```python
from build123d import *

# Parameters (mm, degrees)
SKETCH1_R                = 27.5
SKETCH1_R_2              = 2.5
BOSS_EXTRUDE1_DEPTH      = 10.5
SKETCH2_R                = 4
SKETCH2_R_2              = 2.5
BOSS_EXTRUDE2_DEPTH      = 11
SKETCH3_R                = 5
SKETCH3_R_2              = 4
BOSS_EXTRUDE3_DEPTH      = 1.5
BOSS_EXTRUDE4_DEPTH      = 11
FILLET2_R                = 0.5
FILLET5_R                = 1.5
CIRPATTERN1_COUNT        = 3
FILLET2_OF_CIRPATTERN1_R = 0.5
FILLET5_OF_CIRPATTERN1_R = 1.5
SKETCH5_R                = 1.5
CUT_EXTRUDE1_DEPTH       = 45.438159278
SKETCH6_R                = 2.75
CUT_EXTRUDE2_DEPTH       = 3
SKETCH7_R                = 4.25
CUT_EXTRUDE3_DEPTH       = 5
CIRPATTERN2_COUNT        = 3
CHAMFER1_SIZE            = 0.5
SKETCH9_R                = 8
CUT_EXTRUDE4_DEPTH       = 41.416580756
BOSS_EXTRUDE7_START      = -5.5
SKETCH10_R               = 8
SKETCH10_R_2             = 6.5
BOSS_EXTRUDE7_DEPTH      = 5.5
CHAMFER2_SIZE            = 0.5
BOSS_EXTRUDE8_START      = -1.5
SKETCH11_R               = 29
SKETCH11_R_2             = 27.5
BOSS_EXTRUDE8_DEPTH      = 1.5


with BuildPart() as part:
    # Sketch1 → Boss-Extrude1 (new body)
    with BuildSketch(Plane.XY):
        with Locations(Location((0, 0, 0), (0, 0, 180))):
            Circle(SKETCH1_R)
        with Locations(Location((0, 22.05, 0), (0, 0, 180))):
            Circle(SKETCH1_R_2, mode=Mode.SUBTRACT)
        with Locations(Location((19.095860153, -11.025, 0), (0, 0, 180))):
            Circle(SKETCH1_R_2, mode=Mode.SUBTRACT)
        with Locations(Location((-19.095860153, -11.025, 0), (0, 0, 180))):
            Circle(SKETCH1_R_2, mode=Mode.SUBTRACT)
    extrude(amount=BOSS_EXTRUDE1_DEPTH)

    # Sketch2 → Boss-Extrude2 (add)
    with BuildSketch(Plane.XY.offset(10.5)):
        with Locations((0, 22.05)):
            Circle(SKETCH2_R)
        with Locations(Location((0, 22.05, 0), (0, 0, 180))):
            Circle(SKETCH2_R_2, mode=Mode.SUBTRACT)
    boss_extrude2 = extrude(amount=BOSS_EXTRUDE2_DEPTH)

    # Sketch3 → Boss-Extrude3 (add)
    with BuildSketch(Plane.XY.offset(10.5)):
        with Locations((0, 22.05)):
            Circle(SKETCH3_R)
        with Locations((0, 22.05)):
            Circle(SKETCH3_R_2, mode=Mode.SUBTRACT)
    boss_extrude3 = extrude(amount=BOSS_EXTRUDE3_DEPTH)

    # Sketch4 → Boss-Extrude4 (add)
    with BuildSketch(Plane.XY.offset(10.5)):
        with BuildLine():
            ThreePointArc((-8.731428479, 7.173015873), (-14.812140242, 13.209015809), (-17.238712835, 21.426077098))
            ThreePointArc((-17.238712835, 21.426077098), (-23.815698604, 13.75), (-27.174883487, 4.216124695))
            ThreePointArc((-27.174883487, 4.216124695), (-18.845413371, 6.223181829), (-10.577728207, 3.975130938))
            ThreePointArc((-10.577728207, 3.975130938), (-9.786087063, 5.65), (-8.731428479, 7.173015873))
        make_face()
    boss_extrude4 = extrude(amount=BOSS_EXTRUDE4_DEPTH)

    # Fillet2
    fillet2_edges = [part.edges().sort_by_distance(p)[0] for p in [
        (-5, 22.05, 12),
    ]]
    fillet(fillet2_edges, radius=FILLET2_R)

    # Fillet5
    # the kernel refuses this fillet: 1.5 mm, written as the material it takes off along each edge
    with BuildSketch(Plane(origin=(-17.238712835, 21.426077098, 10.5), x_dir=(0.11627707658946446, -0.9932168149300573, 0), z_dir=(0, 0, 1))) as fillet5_piece_1:
        with BuildLine():
            CenterArc((2.88996817, -1.495158903), FILLET5_R, 94.604481761, 123.727317632)
            ThreePointArc((1.713319765, -2.425480639), (0.8238966, -1.235883765), (0, 0))
            ThreePointArc((0, 0), (1.384776415, -0.055672613), (2.769552829, 0))
        make_face()
    extrude(amount=18.423956554, mode=Mode.SUBTRACT)
    with BuildSketch(Plane(origin=(-27.174883487, 4.216124695, 10.5), x_dir=(0.9182895314900276, 0.39590950526076735, 0), z_dir=(0, 0, 1))) as fillet5_piece_2:
        with BuildLine():
            CenterArc((2.88996817, 1.495158903), FILLET5_R, 141.668200607, 123.727317632)
            ThreePointArc((1.713319765, 2.425480639), (0.8238966, 1.235883765), (0, 0))
            ThreePointArc((0, 0), (1.384776415, 0.055672613), (2.769552829, 0))
        make_face()
    extrude(amount=18.423956554, mode=Mode.SUBTRACT)
    with BuildSketch(Plane(origin=(-10.577728207, 3.975130938, 10.5), x_dir=(-0.8902885516550605, 0.4553968541743943, 0), z_dir=(0, 0, 1))) as fillet5_piece_3:
        with BuildLine():
            CenterArc((1.570607816, -1.498571769), FILLET5_R, 92.500493645, 86.512353367)
            ThreePointArc((0.070830441, -1.472729442), (0.059461178, -0.735208239), (0, 0))
            ThreePointArc((0, 0), (0.752582912, -0.016424661), (1.505165824, 0))
        make_face()
    extrude(amount=14.762914559, mode=Mode.SUBTRACT)
    with BuildSketch(Plane(origin=(-8.731428479, 7.173015873, 10.5), x_dir=(-0.5830170750372249, -0.8124599006812822, 0), z_dir=(0, 0, 1))) as fillet5_piece_4:
        with BuildLine():
            CenterArc((1.572292256, -1.496804369), FILLET5_R, 93.740653048, 86.512353367)
            ThreePointArc((0.07230688, -1.50342804), (0.052559138, -0.750924993), (0, 0))
            ThreePointArc((0, 0), (0.737215871, -0.024073752), (1.474431742, 0))
        make_face()
    extrude(amount=14.762914559, mode=Mode.SUBTRACT)

    # CirPattern1: Boss-Extrude2, Boss-Extrude3, Boss-Extrude4 ×3 about axis
    cirpattern1_axis = Axis((0, 0, 0), (0, 0, 1))
    add([boss_extrude2.rotate(cirpattern1_axis, i * 360 / CIRPATTERN1_COUNT) for i in range(1, CIRPATTERN1_COUNT)])
    add([boss_extrude3.rotate(cirpattern1_axis, i * 360 / CIRPATTERN1_COUNT) for i in range(1, CIRPATTERN1_COUNT)])
    add([boss_extrude4.rotate(cirpattern1_axis, i * 360 / CIRPATTERN1_COUNT) for i in range(1, CIRPATTERN1_COUNT)])

    # Fillet2 of CirPattern1
    fillet2_of_cirpattern1_edges = [part.edges().sort_by_distance(p)[0] for p in [
        (-16.595860153, -15.355127019, 12),
        (21.595860153, -6.694872981, 12),
    ]]
    fillet(fillet2_of_cirpattern1_edges, radius=FILLET2_OF_CIRPATTERN1_R)

    # Fillet5 of CirPattern1
    # the kernel refuses this fillet: 1.5 mm, written as the material it takes off along each edge
    with BuildSketch(Plane(origin=(-9.936170652, -25.642201793, 10.5), x_dir=(0.950591872836604, -0.31044337856845616, 0), z_dir=(0, 0, 1))) as fillet5_of_cirpattern1_piece_1:
        with BuildLine():
            CenterArc((2.888594005, 1.497812019), FILLET5_OF_CIRPATTERN1_R, 149.367724673, 123.727317632)
            ThreePointArc((1.597911292, 2.262101319), (0.844427641, 1.098929988), (0, 0))
            ThreePointArc((0, 0), (1.484791311, -0.040112987), (2.969582622, 0))
        make_face()
    extrude(amount=18.423956554, mode=Mode.SUBTRACT)
    with BuildSketch(Plane(origin=(9.936170652, -25.642201793, 10.5), x_dir=(-0.9505918728365876, -0.31044337856850573, 0), z_dir=(0, 0, 1))) as fillet5_of_cirpattern1_piece_2:
        with BuildLine():
            CenterArc((2.888594005, -1.497812019), FILLET5_OF_CIRPATTERN1_R, 86.904957695, 123.727317632)
            ThreePointArc((1.597911292, -2.262101319), (0.844427641, -1.098929988), (0, 0))
            ThreePointArc((0, 0), (1.484791311, 0.040112987), (2.969582622, 0))
        make_face()
    extrude(amount=18.423956554, mode=Mode.SUBTRACT)
    with BuildSketch(Plane(origin=(1.846299728, -11.148146811, 10.5), x_dir=(0.050759031308987616, -0.998710929518934, 0), z_dir=(0, 0, 1)), Plane(origin=(8.731428479, 7.173015873, 10.5), x_dir=(0.8395295203460723, 0.5433140753445413, 0), z_dir=(0, 0, 1))) as fillet5_of_cirpattern1_piece_3:
        with BuildLine():
            CenterArc((1.570607816, -1.498571769), FILLET5_OF_CIRPATTERN1_R, 92.500493645, 86.512353367)
            ThreePointArc((0.070830441, -1.472729442), (0.059461178, -0.735208239), (0, 0))
            ThreePointArc((0, 0), (0.752582912, -0.016424661), (1.505165824, 0))
        make_face()
    extrude(amount=14.762914559, mode=Mode.SUBTRACT)
    with BuildSketch(Plane(origin=(-1.846299728, -11.148146811, 10.5), x_dir=(0.9951194510647849, -0.09867764748169308, 0), z_dir=(0, 0, 1)), Plane(origin=(10.577728207, 3.975130938, 10.5), x_dir=(-0.41210237602756, 0.9111375481629761, 0), z_dir=(0, 0, 1))) as fillet5_of_cirpattern1_piece_4:
        with BuildLine():
            CenterArc((1.572292256, -1.496804369), FILLET5_OF_CIRPATTERN1_R, 93.740653048, 86.512353367)
            ThreePointArc((0.07230688, -1.50342804), (0.052559138, -0.750924993), (0, 0))
            ThreePointArc((0, 0), (0.737215871, -0.024073752), (1.474431742, 0))
        make_face()
    extrude(amount=14.762914559, mode=Mode.SUBTRACT)
    with BuildSketch(Plane(origin=(27.174883487, 4.216124695, 10.5), x_dir=(-0.918289531490027, 0.3959095052607686, 0), z_dir=(0, 0, 1))) as fillet5_of_cirpattern1_piece_5:
        with BuildLine():
            CenterArc((2.88996817, -1.495158903), FILLET5_OF_CIRPATTERN1_R, 94.604481761, 123.727317632)
            ThreePointArc((1.713319765, -2.425480639), (0.8238966, -1.235883765), (0, 0))
            ThreePointArc((0, 0), (1.384776415, -0.055672613), (2.769552829, 0))
        make_face()
    extrude(amount=18.423956554, mode=Mode.SUBTRACT)
    with BuildSketch(Plane(origin=(17.238712835, 21.426077098, 10.5), x_dir=(-0.11627707658945366, -0.9932168149300585, 0), z_dir=(0, 0, 1))) as fillet5_of_cirpattern1_piece_6:
        with BuildLine():
            CenterArc((2.88996817, 1.495158903), FILLET5_OF_CIRPATTERN1_R, 141.668200607, 123.727317632)
            ThreePointArc((1.713319765, 2.425480639), (0.8238966, 1.235883765), (0, 0))
            ThreePointArc((0, 0), (1.384776415, 0.055672613), (2.769552829, 0))
        make_face()
    extrude(amount=18.423956554, mode=Mode.SUBTRACT)

    # Sketch5 → Cut-Extrude1 (cut, through all)
    with BuildSketch(Plane.XY.offset(21.5)):
        with Locations((-20.351596989, 11.75)):
            Circle(SKETCH5_R)
    cut_extrude1 = extrude(amount=-CUT_EXTRUDE1_DEPTH, mode=Mode.SUBTRACT)

    # Sketch6 → Cut-Extrude2 (cut)
    with BuildSketch(Plane(origin=(0, 0, 0), x_dir=(-1, 0, 0), z_dir=(0, 0, -1))):
        with Locations((20.351596989, 11.75)):
            Circle(SKETCH6_R)
    cut_extrude2 = extrude(amount=-CUT_EXTRUDE2_DEPTH, mode=Mode.SUBTRACT)

    # Sketch7 → Cut-Extrude3 (cut)
    with BuildSketch(Plane(origin=(0, 0, 0), x_dir=(-1, 0, 0), z_dir=(0, 0, -1))):
        with Locations((0, 22.05)):
            Circle(SKETCH7_R)
    cut_extrude3 = extrude(amount=-CUT_EXTRUDE3_DEPTH, mode=Mode.SUBTRACT)

    # CirPattern2: Cut-Extrude1, Cut-Extrude2, Cut-Extrude3 ×3 about axis
    cirpattern2_axis = Axis((0, 0, 0), (0, 0, 1))
    add([cut_extrude1.rotate(cirpattern2_axis, i * 360 / CIRPATTERN2_COUNT) for i in range(1, CIRPATTERN2_COUNT)], mode=Mode.SUBTRACT)
    add([cut_extrude2.rotate(cirpattern2_axis, i * 360 / CIRPATTERN2_COUNT) for i in range(1, CIRPATTERN2_COUNT)], mode=Mode.SUBTRACT)
    add([cut_extrude3.rotate(cirpattern2_axis, i * 360 / CIRPATTERN2_COUNT) for i in range(1, CIRPATTERN2_COUNT)], mode=Mode.SUBTRACT)

    # Chamfer1
    chamfer1_edges = [part.edges().sort_by_distance(p)[0] for p in [
        (27.5, 0, 0),
    ]]
    chamfer(chamfer1_edges, length=CHAMFER1_SIZE)

    # Sketch9 → Cut-Extrude4 (cut, through all)
    with BuildSketch(Plane.XY.offset(10.5)):
        Circle(SKETCH9_R)
    extrude(amount=-CUT_EXTRUDE4_DEPTH, mode=Mode.SUBTRACT)

    # Sketch10 → Boss-Extrude7 (add)
    with BuildSketch(Plane(origin=(0, 0, 0), x_dir=(-1, 0, 0), z_dir=(0, 0, -1)).offset(BOSS_EXTRUDE7_START)):
        with Locations(Location((0, 0, 0), (0, 0, 180))):
            Circle(SKETCH10_R)
        Circle(SKETCH10_R_2, mode=Mode.SUBTRACT)
    extrude(amount=BOSS_EXTRUDE7_DEPTH)

    # Chamfer2
    chamfer2_edges = [part.edges().sort_by_distance(p)[0] for p in [
        (-8, 0, 10.5),
    ]]
    chamfer(chamfer2_edges, length=CHAMFER2_SIZE)

    # Sketch11 → Boss-Extrude8 (add)
    with BuildSketch(Plane.XY.offset(10.5).offset(BOSS_EXTRUDE8_START)):
        Circle(SKETCH11_R)
        with Locations(Location((0, 0, 0), (0, 0, 180))):
            Circle(SKETCH11_R_2, mode=Mode.SUBTRACT)
    extrude(amount=BOSS_EXTRUDE8_DEPTH)


solid = part.part
```
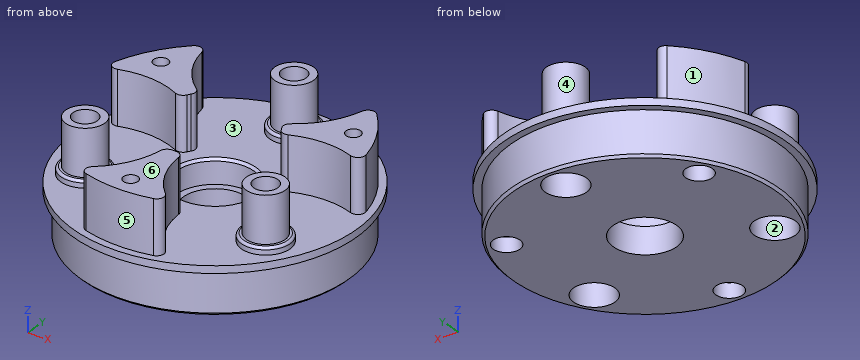
Work out the finished part from the listing and answer in its coordinate system (mm). Face numbers are marked on the shaded views. A direction names the side the tool comes from. Coordinates: 2 decimals unless noted, no trailing zeros. Write each loop counter-clockwise with the first axis right and the second up, starting at its lowest first coordinate (ties: lowest second). Pieces come first, ordered by that corner, then holes. Notation, with made-up numbers: (59, -23) - (100, -23) arc R32 ccw to (100, 15) - close; hole circle Ø4 at (0.5, -3.75). An arc over 180 degrees is marked (long way). Answer as a JSON object with one key per item and string values.
Q1. Find section B-B (z = 17.75). State how many separate pieces and enclosed holes the cut face has, plus the area to 3 significant figures.
Results list:
{"separate pieces": "6", "enclosed holes": "6", "area": "499 mm^2"}
Q2. Consider L1, parallel to Y at x = 0, z = 7.6; L2, parallel to Y at x = 0, z = 10; L3, parallel to X at y = 12.5, z = 5.5. Determine where each line is inside the solid, lowest interval first. Write a range as from..to.
Results list:
{"L1": "y = -27.5..-25, -22..-8, 8..19.55, 24.55..27.5", "L2": "y = -29..-25, -22..-8, 8..19.55, 24.55..29", "L3": "x = -24.49..-21.65, -19.05..19.05, 21.65..24.49"}
Q3. Find section A-A (y = 0). Write down the section's boundary in (x, z), plus the area to 3 significant figures.
Results list:
{"outline": "(-29, 9) - (-27.5, 9) - (-27.5, 0.5) - (-27, 0) - (-6.5, 0) - (-6.5, 5.5) - (-8, 5.5) - (-8, 10) - (-8.5, 10.5) - (-29, 10.5) - close; (6.5, 0) - (27, 0) - (27.5, 0.5) - (27.5, 9) - (29, 9) - (29, 10.5) - (8.5, 10.5) - (8, 10) - (8, 5.5) - (6.5, 5.5) - close", "area": "430 mm^2"}
Q4. Given pin 1 Ø12 at (y, z) = (1, 17) entering from -X; pin 2 Ø10 at (x, y) = (0, 22.05) entering from -Z; pin 3 Ø12 at (x, z) = (-16.5, 2.5) entering from +Y; pin 4 Ø4.5 at (x, y) = (19.1, -11.02) entering from -Z, each flat-ended and moving along its own axis, determine where each tip first touches the part or whether it passes through.
Results list:
{"pin 1": "stops at x = -26.61", "pin 2": "stops at z = 0", "pin 3": "stops at y = 25.42", "pin 4": "passes through"}
Q5. For a pull along X with two mould halves and no side action, classify the marked faces 4, 5 and 6 as pulls with the +X half, pulls with the -X half, needs draft (parallel to the pull), parting line crosses it, or undercut.
Results list:
{"face 4": "undercut", "face 5": "parting line crosses it", "face 6": "needs draft"}
Q6. Which of the six approach directions +Z, -Z, +X, -X, +Y, -Y give full straight-line access (tool end or side, diameter ignored) to the marked faces 1, 2 and 3?
Results list:
{"face 1": "+Z, -X, +Y", "face 2": "-Z", "face 3": "+Z"}
